Build history of the part. All positions in model axes, mm. Face numbers are marked on the shaded views. Give positions to 0.01 mm unless a question says otherwise; leave off trailing zeros. Write each loop counter-clockwise with the first axis right and the second up, starting at its lowest first coordinate (ties: lowest second). Pieces come first, ordered by that corner, then holes. Notation, with made-up numbers: (26.5, -9.5) -> (54.5, -9.5) arc R22 cw to (54.5, 28.5) -> close; hole circle Ø8 at (65, 80). An arc over 180 degrees is marked (long way). One line per question, with ' | ' between items. Start each with the question number.
(1) Band-saw the part on A-A, the plane y = -19.5. Give the cut face in (x, z).
(2) Band-saw the part on B-B, the plane x = 10. Give the cut face in (y, z).
(3) Band-saw the part on C-C, the plane x = -12. Give the cut face in (y, z).
(4) Pull direction X, two halves, no side cores. Call the marked faces 1 and 2: released by +X, released by -X, zero draft, split by the parting line, or undercut.
(5) Pin check, flat tips, straight feed: P1, Ø12, axis at x = -2.5, z = -1.5, coming from the +Y side; P2, Ø1.5, axis at y = -15.5, z = -15, coming from the -X side; P3, Ø12, axis at x = 9, z = -2, coming from the +Y side; P4, Ø2.5, axis at x = -14.5, y = -23, coming from the -Z side. Stop position of each tip, or through.
(6) Drill centre lines: probe 1 along Z at (x, y) = (0, -12); probe 2 along X at (y, z) = (-18.75, -10); probe 3 along Y at (x, z) = (0, 20.6) (3 decimals). Where is each one in solid material? Low to high. Write a range as from..to.
Autodesk Inventor part; units mm, degrees
ref_plane "YZ Plane" through (0, 0, 0) normal (1, 0, 0) x (0, 1, 0)
ref_plane "XZ Plane" through (0, 0, 0) normal (0, 1, 0) x (-1, 0, 0)
ref_plane "XY Plane" through (0, 0, 0) normal (0, 0, 1) x (1, 0, 0)
sketch "Sketch2" plane through (0, 0, 0) normal (0, 0, 1) x (1, 0, 0)
  circle A0 centre (0, 0) radius 25
  circle A1 centre (0, 0) radius 24
  line L0 (-28.1544, -15) -> (30.7149, -15)
  line L1 (0, -25) -> (0, -24)
  point P0 (20, -15)
  point P1 (18.735, -15)
  dimension "d3" = 50
  dimension "d4" = 48
  dimension "d6" = 10
revolve "Revolution1" add sketch "Sketch2" angle 360 about axis through (0, -25, 0) along (0, 1, 0) picked at (16.5634, -17.6598) contours A0 L1 A1 L0
sketch "Sketch3" plane through (0, 0, 0) normal (0, 0, 1) x (1, 0, 0)
  arc A0 (-20, -15) -> (20, -15) centre (0, 0) ccw
  circle A1 centre (0, 0) radius 25
  circle A2 centre (0, 0) radius 25.875
  line L0 (20, -15) -> (21.0835, -15)
  line L1 (-20, -15) -> (20, -15)
  line L2 (0, -15) -> (0, -25)
  line L3 (-20, -15) -> (-21.0835, -15)
  line L4 (0, -25.875) -> (0, -25)
  line L5 (-38.5, 0) -> (38.5, 0)
  line L6 (0, -38.5) -> (0, 38.5)
  point P0 (20, -15)
  dimension "d7" = 51.75
revolve "Revolution2" add sketch "Sketch3" angle 360 about axis through (0, -10, 0) along (0, 1, 0) contours A0 L0 A2 L4
sketch "Sketch4" plane through (0, 0, 0) normal (0, 0, 1) x (1, 0, 0)
  line L0 (19.6202, -16.869) -> (18.4509, -16.869)
  line L1 (0, -25.875) -> (0, -25)
  line L2 (1.3306, -24.9646) -> (1.3306, -25.8408)
  line L3 (-19.6202, -16.869) -> (-18.4509, -16.869)
  line L4 (-1.3306, -24.9646) -> (-1.3306, -25.8408)
  circle A0 centre (0, 0) radius 25
  circle A1 centre (0, 0) radius 25.875
  line L5 (0, -36.225) -> (0, 36.225)
revolve "Revolution4" cut sketch "Sketch4" angle 80 about axis through (0, -10, 0) along (0, -1, 0) contours A1 L2 A0 L0
pattern_circular "Circular Pattern2" count 4 over 360 about axis through (0, -10, 0) along (0, 1, 0) of "Revolution4"
sketch "Sketch6" plane through (0, -15, 0) normal (0, 1, 0) x (1, 0, 0)
  line L0 (-19.6202, 0) -> (-1.3306, 0)
  circle A0 centre (0, 0) radius 19.6202
  circle A1 centre (0, 0) radius 21.0835
  circle A2 centre (0, 0) radius 21.0835
extrude "Extrusion3" add sketch "Sketch6" along normal blind 5
sketch "Sketch7" plane through (0, 0, 0) normal (0, 0, 1) x (1, 0, 0)
  line L0 (-21.0835, -15) -> (21.0835, -15)
  circle A0 centre (0, -13) radius 0.375
  point P0 (0, 0)
  dimension "d24" = 0.75
  dimension "d26" = 2
extrude "Extrusion4" cut sketch "Sketch7" against normal through all
pattern_circular "Circular Pattern3" count 6 over 360 about axis through (0, -10, 0) along (0, 1, 0) of "Extrusion4"
properties part number "Main Mirror"
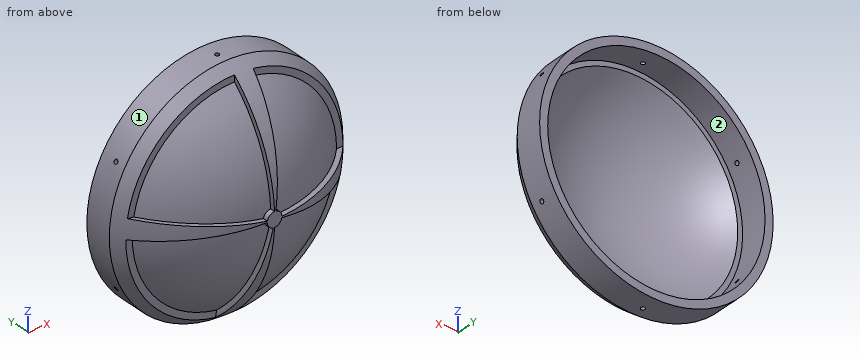
Results:
1) outline: (-17.01, 0) -> (-15.64, 0) arc R15.64 ccw to (-2.72, -15.41) -> (-2.95, -16.75) arc R17.01 ccw to (0, -17.01) -> (0, -15.64) arc R15.64 ccw to (15.41, -2.72) -> (16.75, -2.95) arc R17.01 ccw to (17.01, 0) -> (15.64, 0) arc R15.64 ccw to (2.72, 15.41) -> (2.95, 16.75) arc R17.01 ccw to (0, 17.01) -> (0, 15.64) arc R15.64 ccw to (-15.41, 2.72) -> (-16.75, 2.95) arc R17.01 ccw to start; hole circle Ø27.98 at (0, 0)
2) outline: (-23.86, 0) arc R23.86 ccw to (-23.8, -1.76) -> (-22.84, -1.76) arc R22.91 ccw to (-16.87, -15.51) -> (-16.87, -16.88) arc R23.86 ccw to (-15, -18.56) -> (-10, -18.56) -> (-10, -16.88) -> (-15, -16.88) -> (-15, -15.84) arc R21.82 cw to (-15, 15.84) -> (-15, 16.88) -> (-10, 16.88) -> (-10, 18.56) -> (-15, 18.56) arc R23.86 ccw to (-16.87, 16.88) -> (-16.87, 15.51) arc R22.91 ccw to (-22.91, 0) -> close
3) outline: (-22.92, 0) -> (-21.93, 0) arc R21.93 ccw to (-16.87, -14.02) -> (-16.87, -15.52) arc R22.92 ccw to (-15, -17.34) -> (-10, -17.34) -> (-10, -15.52) -> (-15, -15.52) -> (-15, -14.39) arc R20.78 cw to (-15, 14.39) -> (-15, 15.52) -> (-10, 15.52) -> (-10, 17.34) -> (-15, 17.34) arc R22.92 ccw to (-16.87, 15.52) -> (-16.87, 14.02) arc R21.93 ccw to (-21.83, 2.12) -> (-22.83, 2.12) arc R22.92 ccw to start
4) face 1: split by the parting line | face 2: undercut
5) P1: stops at y = -22.28 | P2: stops at x = -15.36 | P3: stops at y = -18.56 | P4: passes through
6) probe 1: z = -21.08..-19.62, 19.62..21.08 | probe 2: x = -13.17..-11.16, 11.16..13.17 | probe 3: y = -15.657..-13.375, -12.625..-10
